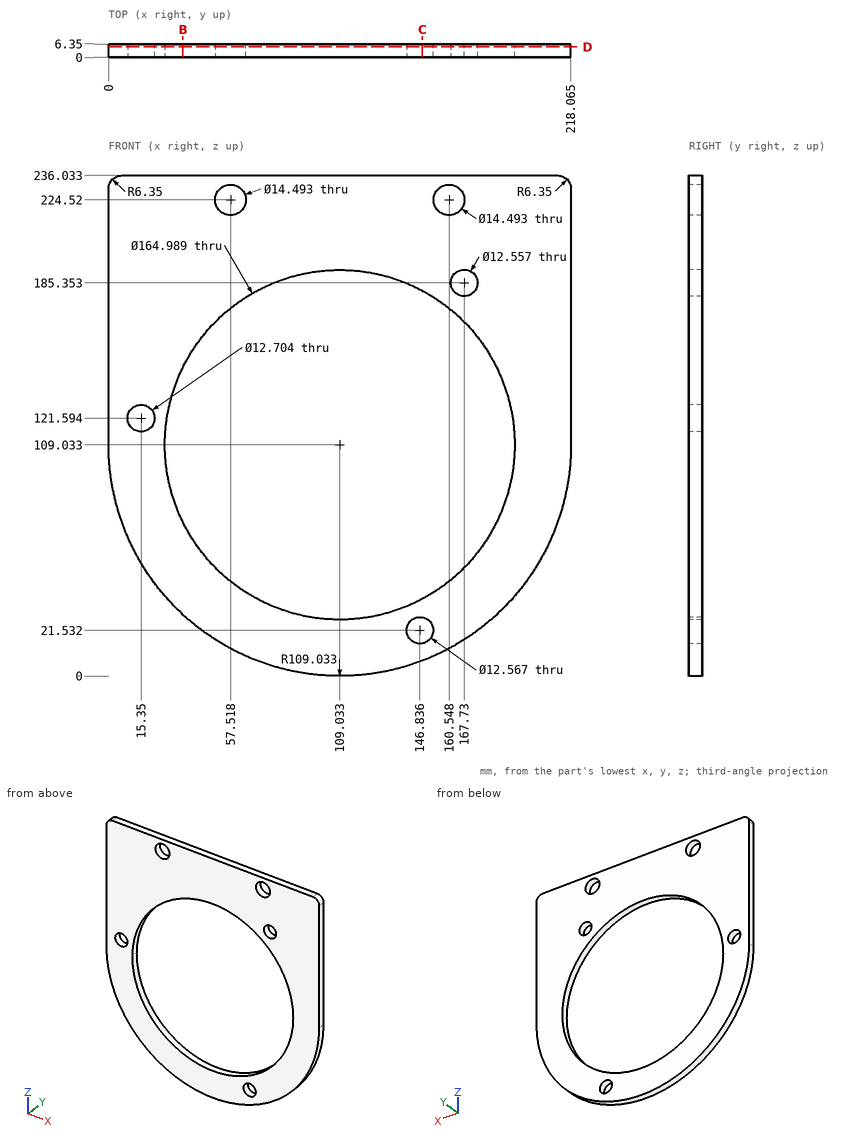
Here's the drawing with two shaded views (mm, measured from the low corner). I have some questions. Round coordinates to 2 decimals unless told otherwise and drop trailing zeros. Order: outer loops, then holes, each group sorted by start corner. A loop starts at its lowest first (then second) coordinate and runs counter-clockwise, first axis right, second up. Notation, with made-up numbers: (58.5, 68) -> (100.5, 68) arc R19 cw to (100.5, 90) -> close; hole circle Ø7 at (-1, 84.5). An arc over 180 degrees is marked (long way). Write each question's results on one line, items separated by ' | '. Start each with the question number.
Item 1: If we section it at D-D, the plane y = 5: State how many separate pieces and enclosed holes the cut face has, then the cut area to 3 significant figures.
Item 2: Will this pin go through, and if not, where does the flat tip stop? pin 1 (2 mm diameter, centred on x = 45, y = 3, fed in from -Z) (1 decimal).
Item 3: Please list where these lines run through material, in increasing order: L1, parallel to Z at x = 61.5, y = 4 (1 decimal); L2, parallel to X at y = 3.75, z = 224 (1 decimal); L3, parallel to X at y = 4.75, z = 121 (1 decimal).
Item 4: If we section it at C-C, the plane x = 148: Write out the boundary of the cut face in (y, z).
Item 5: If we section it at B-B, the plane x = 35: Write out the boundary of the cut face in (y, z).
Results:
1) separate pieces: 1 | enclosed holes: 6 | area: 24,300 mm2
2) pin 1: stops at z = 20.1
3) L1: z = 10.9 to 41.6, 176.5 to 218.5, 230.6 to 236 | L2: x = 0 to 50.3, 64.7 to 153.3, 167.8 to 218.1 | L3: x = 0 to 9, 21.7 to 27.4, 190.7 to 218.1
4) outline: (0, 7.2) -> (6.35, 7.2) -> (6.35, 15.36) -> (0, 15.36) -> close; (0, 27.71) -> (6.35, 27.71) -> (6.35, 36.32) -> (0, 36.32) -> close; (0, 181.74) -> (6.35, 181.74) -> (6.35, 236.03) -> (0, 236.03) -> close
5) outline: (0, 28.99) -> (6.35, 28.99) -> (6.35, 72.64) -> (0, 72.64) -> close; (0, 145.43) -> (6.35, 145.43) -> (6.35, 236.03) -> (0, 236.03) -> close
